Solid Edge part; units mm, degrees
sketch "Sketch1" plane through (0, 0, 0) normal (0, 0, 1) x (1, 0, 0)
  circle A0 centre (0, 0) radius 25
extrude "Protrusion1" add sketch "Sketch1" against normal blind 8
sketch "Sketch2" plane through (0, 0, 0) normal (0, 0, 1) x (1, 0, 0)
  circle A0 centre (0, 0) radius 18
extrude "BigHole" cut sketch "Sketch2" against normal blind 4
sketch "Sketch3" plane through (0, 0, -4) normal (0, 0, 1) x (1, 0, 0)
  circle A0 centre (0, 0) radius 4
extrude "SmallMiddleHoleP1" cut sketch "Sketch3" against normal blind 6
sketch "Sketch4" plane through (0, 0, -8) normal (0, 0, -1) x (1, 0, 0)
  circle A0 centre (0, 0) radius 6
extrude "SmallExtensionBottom" add sketch "Sketch4" along normal blind 2
sketch "Sketch5" plane through (0, 0, -10) normal (0, 0, -1) x (0, -1, 0)
  circle A0 centre (0, 0) radius 4
extrude "SmallMiddleHoleP2" cut sketch "Sketch5" against normal blind 2
sketch "Sketch6" plane through (0, 0, -4) normal (0, 0, 1) x (1, 0, 0)
  circle A0 centre (12, 0) radius 5
  circle A1 centre (-12, 0) radius 5
  circle A2 centre (0, 12) radius 5
  circle A3 centre (0, -12) radius 5
extrude "v_2HolesLR" cut sketch "Sketch6" against normal blind 6
Verification items for the finished model (mm, model axes). A direction names the side the tool comes from. Round coordinates to 2 decimals unless told otherwise and drop trailing zeros. Order: outer loops, then holes, each group sorted by start corner. A loop starts at its lowest first (then second) coordinate and runs counter-clockwise, first axis right, second up. Notation, with made-up numbers: (34.5, -31) -> (72.5, -31) arc R22 ccw to (72.5, -9) -> close; hole circle Ø11 at (7, 11). An arc over 180 degrees is marked (long way). Put each result on its own line as item: value.
1) Section check C-C (x = -16). Record the cut outline in (y, z), then the cut area to 3 significant figures.
Final values:
outline: (-19.21, -8) -> (-3, -8) -> (-3, -4) -> (-8.25, -4) -> (-8.25, 0) -> (-19.21, 0) -> close; (3, -8) -> (19.21, -8) -> (19.21, 0) -> (8.25, 0) -> (8.25, -4) -> (3, -4) -> close
area: 217 mm^2
2) Depth check by flat-ended pin: pin 1 (2 mm diameter, centred on x = 14.5, y = 5, fed in from -Z); pin 2 (21.5 mm diameter, centred on x = 0, y = 0, fed in from +Z); pin 3 (6 mm diameter, centred on x = -6, z = -5.5, fed in from +Y). Enter the tip coordinate at first touch or a pass-through.
Final values:
pin 1: stops at z = -8
pin 2: stops at z = -4
pin 3: stops at y = 24.82
3) Material ranges on line 1 (Y direction, x = 0, z = -6); line 2 (X direction, y = 0, z = -9.55); line 3 (Z direction, x = -6.5, y = 14.5), recorded low to high.
Final values:
line 1: y = -25 to -17, -7 to -4, 4 to 7, 17 to 25
line 2: x = -6 to -4, 4 to 6
line 3: z = -8 to -4
4) Section check D-D (z = -5.25). Record the cut outline in (x, y), then the cut area to 3 significant figures.
Final values:
outline: circle Ø50 at (0, 0); hole circle Ø10 at (-12, 0); hole circle Ø10 at (0, -12); hole circle Ø10 at (0, 12); hole circle Ø8 at (0, 0); hole circle Ø10 at (12, 0)
area: 1,600 mm^2
5) Section check A-A (x = 0). Record the cut outline in (y, z), then the cut area to 3 significant figures.
Final values:
outline: (-25, -8) -> (-17, -8) -> (-17, -4) -> (-18, -4) -> (-18, 0) -> (-25, 0) -> close; (-7, -8) -> (-6, -8) -> (-6, -10) -> (-4, -10) -> (-4, -4) -> (-7, -4) -> close; (4, -10) -> (6, -10) -> (6, -8) -> (7, -8) -> (7, -4) -> (4, -4) -> close; (17, -8) -> (25, -8) -> (25, 0) -> (18, 0) -> (18, -4) -> (17, -4) -> close
area: 152 mm^2
6) Set-up check for faces 4 (the cylindrical face through (-2.343, 17.847, -1.972)), 5 (the cylindrical face through (16.77, 1.5, -5.97)): record each of +Z, -Z, +X, -X, +Y, -Y from which the full face is reachable in a straight line by a thin tool's end or side.
Final values:
face 4: +Z
face 5: +Z, -Z
7) Section check B-B (y = 11). Record the cut outline in (x, z), then the cut area to 3 significant figures.
Final values:
outline: (-22.45, -8) -> (-4.9, -8) -> (-4.9, -4) -> (-14.25, -4) -> (-14.25, 0) -> (-22.45, 0) -> close; (4.9, -8) -> (22.45, -8) -> (22.45, 0) -> (14.25, 0) -> (14.25, -4) -> (4.9, -4) -> close
area: 206 mm^2
8) Mould release check, pull along Y, two halves, no side actions. Record for faces 1 (the flat face through (-4.3, 0.3, -4)), 2 (the flat face through (5, -5, -8)), 3 (the cylindrical face through (-6, 0, -9)): +Y half, -Y half, draft (parallel to the pull), parting line (faces both ways), or undercut.
Final values:
face 1: undercut
face 2: draft
face 3: parting line
